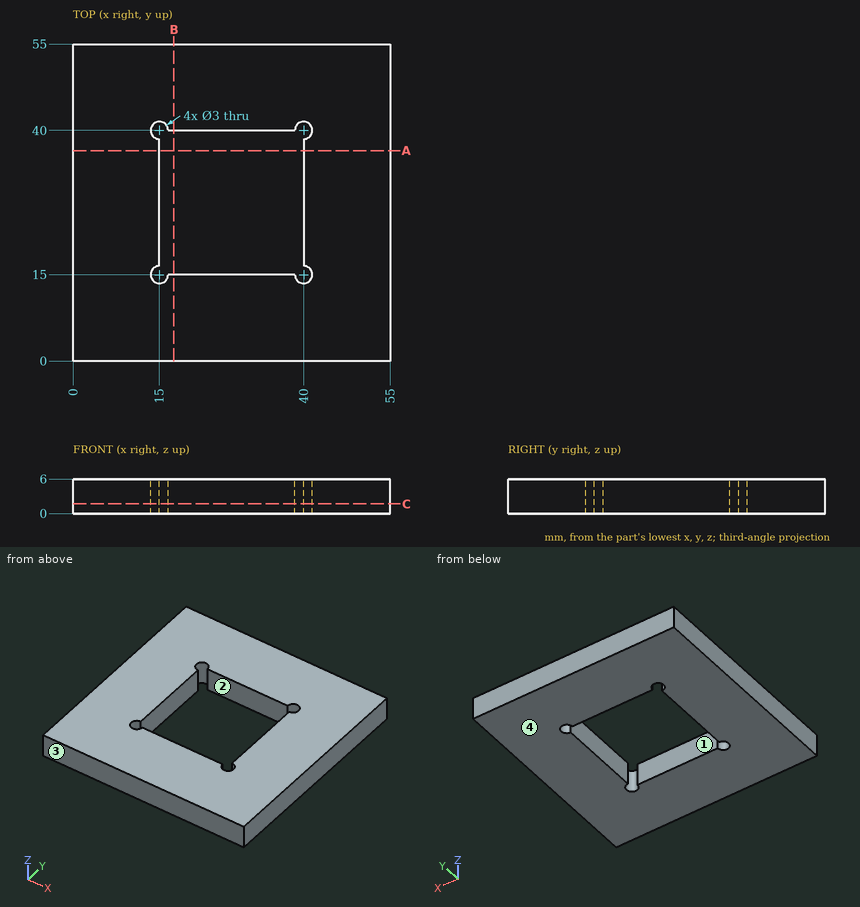
Part print with two shaded views. Sizes in mm from the minimum x, y, z corner. Give positions to 0.01 mm unless a question says otherwise; leave off trailing zeros. Write each loop counter-clockwise with the first axis right and the second up, starting at its lowest first coordinate (ties: lowest second). Pieces come first, ordered by that corner, then holes.
1) Cut at A-A on y = 36.5. Write the cut outline in (x, z), then the cut area to 3 significant figures.
Resolved:
outline: (0, 0) - (15, 0) - (15, 6) - (0, 6) - close; (40, 0) - (55, 0) - (55, 6) - (40, 6) - close
area: 180 mm2
2) Probe L1, parallel to Y at x = 29.5, z = 5.3; L2, parallel to X at y = 14, z = 3.25. List the from-to ranges inside material, lowest first.
Resolved:
L1: y = 0 to 15, 40 to 55
L2: x = 0 to 13.88, 16.12 to 38.88, 41.12 to 55
3) Cut at C-C on z = 1.7. Write the cut outline in (x, y).
Resolved:
outline: (0, 0) - (55, 0) - (55, 55) - (0, 55) - close; hole (15, 16.5) arc R1.5 ccw (long way) to (16.5, 15) - (38.5, 15) arc R1.5 ccw (long way) to (40, 16.5) - (40, 38.5) arc R1.5 ccw (long way) to (38.5, 40) - (16.5, 40) arc R1.5 ccw (long way) to (15, 38.5) - close
4) Two-plate mould, pull along Y, no slides. Class the marked faces 1, 2, 3 and 4: released by +Y, released by -Y, zero draft, split by the parting line, or undercut.
Resolved:
face 1: undercut
face 2: undercut
face 3: released by -Y
face 4: zero draft
5) Pin check, flat tips, straight feed: pin 1 (3.5 mm diameter, centred on x = 15, y = 15, fed in from +Z); pin 2 (1.8 mm diameter, centred on x = 15, y = 40, fed in from +Z). Stop position of each tip, or through.
Resolved:
pin 1: stops at z = 6
pin 2: passes through
